Source: CAD feature listing. Evaluate the final solid. Frame: model axes, mm. Face numbers are marked on the shaded views. A direction names the side the tool comes from. Give positions to 0.01 mm unless a question says otherwise; leave off trailing zeros. Loops run counter-clockwise (first coordinate to the right, second up) from the corner with the lowest first, then second, coordinate; pieces in that order, holes last. Notation, with made-up numbers: (-27, 89.25) - (32, 89.25) arc R29 ccw to (32, 112.25) - close; hole circle Ø7 at (-25.5, 63). An arc over 180 degrees is marked (long way). Write each question's results on one line, items separated by ' | '. Start each with the question number.
(1) Cut plane D-D on z = 0.2. Return the cut outline in (x, y), then the cut area to 3 significant figures.
(2) Material intervals for line 1 along X through (y, z) = (23.25, -0.65); line 2 along Y through (x, z) = (-13, 0.3); line 3 along X through (y, z) = (21.25, 0.05), sorted ascending. Write a range as [from, to].
(3) Reachability of the marked faces 4, 5 and 6 from +Z, -Z, +X, -X, +Y, -Y: full face, straight path, thin tool, end or side. Return the list, or none.
(4) Cut plane A-A on z = -0.75. Return the cut outline in (x, y), then the cut area to 3 significant figures.
(5) Cut plane B-B on y = 25. Return the cut outline in (x, z), then the cut area to 3 significant figures.
(6) Cut plane C-C on x = -11. Return the cut outline in (y, z), then the cut area to 3 significant figures.
(7) Contact query for flat-ended pins moving along their axis: pin 1 (0.6 mm diameter, centred on x = -6.5, z = 0.5, fed in from -Y); pin 2 (4 mm diameter, centred on x = -8, y = 17, fed in from -Z); pin 3 (0.6 mm diameter, centred on y = 25, z = -1, fed in from -X). Output: stop coordinate, or through.
(8) Pull-direction query (X, two-part tool) for the marked faces 1, 2 and 3; classes: pulls with the +X half, pulls with the -X half, needs draft (parallel to the pull), parting line crosses it, or undercut.
Autodesk Fusion 360 part; units mm, degrees
sketch "Sketch1" plane through (0, 22, 0) normal (0, 1, 0) x (-1, 0, 0)
  line L0 (11.5698, 0.25) -> (15.3, 0.25)
  line L1 (15.3, 0.25) -> (15.3, -0.5)
  line L2 (15.3, -0.5) -> (15.6004, -0.5)
  line L3 (15.6004, -0.5) -> (15.6004, -1.2)
  line L4 (15.6004, -1.2) -> (16.0004, -1.2)
  line L5 (16.0004, -1.2) -> (16.0004, -0.5)
  line L6 (16.0004, -0.5) -> (16.3, -0.5)
  line L7 (16.3, -0.5) -> (16.3, 1.05)
  line L8 (16.3, 1.05) -> (5, 1.05)
  line L9 (11.5698, -1.2) -> (11.5698, 0.25)
  line L10 (11.5698, -0.6208) -> (11.2698, -0.6208) construction
  line L11 (11.2698, -0.5) -> (11.2698, -1.2)
  line L12 (11.2698, -0.5) -> (10.5698, -0.5)
  line L13 (10.5698, -0.5) -> (10.5698, -1.2)
  line L14 (10.5698, -0.678) -> (10.2698, -0.678) construction
  line L15 (10.2698, 1.05) -> (10.2698, -1.2)
  line L16 (10.2698, 1.05) -> (16.3, 1.05)
  line L17 (16.3, -0.5) -> (16.0004, -0.5)
  line L18 (16.0004, -1.2) -> (15.6004, -1.2)
  line L19 (15.6004, -0.5) -> (15.3, -0.5)
  line L20 (15.3, 0.25) -> (11.5698, 0.25)
  line L21 (11.5698, -1.2) -> (11.2698, -1.2)
  line L22 (11.5698, -1.2) -> (11.2698, -1.2)
  line L23 (11.2698, -0.5) -> (10.5698, -0.5)
  line L24 (10.5698, -1.2) -> (10.2698, -1.2)
  line L25 (10.2698, 1.05) -> (16.3, 1.05)
  line L26 (16.3, -0.5) -> (16.0004, -0.5)
  line L27 (16.0004, -1.2) -> (15.6004, -1.2)
  line L28 (15.6004, -0.5) -> (15.3, -0.5)
  line L29 (15.3, 0.25) -> (11.5698, 0.25)
  dimension "d14" = 0.3
  dimension "d15" = 0.7
  dimension "d16" = 0.3
extrude "Extrude1" add sketch "Sketch1" along normal blind 8.2 makes body 1
copy_body "Body->Comp1" bodies 1 removing the originals makes body 2 in component "Component"
move_face "OffsetFaces1" offset 0.3 1 faces at (-12.8132, 24.7333, 0.25) on bodies 2 in component "Component"
move_face "OffsetFaces2" offset -0.4 1 faces at (-12.2798, 27.4667, 1.05) on bodies 2 in component "Component"
move_face "OffsetFaces3" offset 3.3 1 faces at (-10.2698, 24.7333, 0.0333) on bodies 2 in component "Component"
move_face "OffsetFaces4" offset -3.3 1 faces at (-10.5698, 24.7333, -0.7333) on bodies 2 in component "Component"
move_face "OffsetFaces5" offset 3.3 1 faces at (-11.2698, 24.7333, -0.7333) on bodies 2 in component "Component"
move_face "OffsetFaces6" offset -3.3 1 faces at (-11.5698, 27.4667, -0.8167) on bodies 2 in component "Component"
move_face "OffsetFaces7" offset -4.2 1 faces at (-10.5132, 22, 0.4167) on bodies 2 in component "Component"
move_face "OffsetFaces8" offset -0.1 1 faces at (-8.2698, 28.8667, -0.4333) on bodies 2 in component "Component"
move_face "OffsetFaces9" offset 0.1 1 faces at (-7.9698, 27.5333, -0.7333) on bodies 2 in component "Component"
move_face "OffsetFaces10" offset 4.255 1 faces at (-10.4798, 26.2, 0.4167) on bodies 2 in component "Component"
move_face "OffsetFaces11" offset 0.3 1 faces at (-6.9698, 24.6967, 0.0333) on bodies 2 in component "Component"
move_face "OffsetFaces12" offset 0.3 1 faces at (-7.8698, 24.6967, -0.7333) on bodies 2 in component "Component"
move_face "OffsetFaces13" offset -0.3 1 faces at (-7.2698, 24.6967, -0.7333) on bodies 2 in component "Component"
move_face "OffsetFaces14" offset -0.3 1 faces at (-8.1698, 24.6967, -0.8167) on bodies 2 in component "Component"
move_face "OffsetFaces15" offset 2.77 1 faces at (-6.6698, 24.6967, 0.0333) on bodies 2 in component "Component"
move_face "OffsetFaces16" offset -2.77 1 faces at (-6.9698, 24.6967, -0.7333) on bodies 2 in component "Component"
move_face "OffsetFaces17" offset 2.77 1 faces at (-7.5698, 24.6967, -0.7333) on bodies 2 in component "Component"
move_face "OffsetFaces18" offset -2.77 1 faces at (-7.8698, 24.6967, -0.8167) on bodies 2 in component "Component"
move_face "OffsetFaces19" offset 6.445 1 faces at (-8.4332, 21.945, 0.4167) on bodies 2 in component "Component"
move_face "OffsetFaces20" offset 1.5 1 faces at (-12.1666, 20.4, 0.65) on bodies 2 in component "Component"
move_face "OffsetFaces21" offset -1.5 1 faces at (-8.4998, 20.4, -0.05) on bodies 2 in component "Component"
sketch "Sketch2" plane through (0, 0, 1.45) normal (0, 0, -1) x (1, 0, 0)
  line L0 (-5.0998, -15.5) -> (-15.3, -15.5)
  line L1 (-15.3, -15.5) -> (-15.3, -30.2)
  line L2 (-15.3, -30.2) -> (-5.0998, -30.2)
  line L3 (-5.0998, -30.2) -> (-5.0998, -15.5)
  line L4 (-5.0998, -15.5) -> (-5.0998, -26.3) construction
  line L5 (-5.0998, -26.3) -> (-15.3, -26.3)
  line L6 (-15.3, -26.3) -> (-15.3, -25.3)
  line L7 (-15.3, -25.3) -> (-5.0998, -25.3)
  line L8 (-5.0998, -25.3) -> (-5.0998, -26.3)
  dimension "d40" = 10.8
  dimension "d41" = 1
extrude "Extrude1'" add sketch "Sketch2" along normal blind 1.5 contours L1 L3 L5 L6 L7 L8 bodies 2 in component "Component"
move_face "OffsetFaces22" offset 6 1 faces at (-11.8999, 25.3, 0.95) on bodies 2 in component "Component"
move_face "OffsetFaces23" offset -6 1 faces at (-8.4998, 26.3, 0.45) on bodies 2 in component "Component"
move_face "OffsetFaces24" offset 0.3 1 faces at (-8.4998, 20.3, 0.45) on bodies 2 in component "Component"
move_face "OffsetFaces25" offset -0.3 1 faces at (-8.4998, 19.3, 0.45) on bodies 2 in component "Component"
move_face "OffsetFaces26" offset -0.6 1 faces at (-8.4998, 19.6, 0.45) on bodies 2 in component "Component"
sketch "Sketch3" plane through (0, 0, 1.45) normal (0, 0, -1) x (1, 0, 0)
  line L0 (-5.0998, -20.6) -> (-15.3, -20.6)
  line L1 (-15.3, -20.6) -> (-15.3, -30.2)
  line L2 (-15.3, -30.2) -> (-5.0998, -30.2)
  line L3 (-5.0998, -30.2) -> (-5.0998, -20.6)
  line L4 (-5.0998, -30.2) -> (-8.3998, -30.2)
  line L5 (-8.3998, -30.2) -> (-8.3998, -29.8)
  line L6 (-8.3998, -29.8) -> (-5.0998, -29.8)
  line L7 (-5.0998, -29.8) -> (-5.0998, -30.2)
  line L8 (-15.3, -30.2) -> (-10.9, -30.2)
  line L9 (-10.9, -30.2) -> (-10.9, -29.8)
  line L10 (-10.9, -29.8) -> (-15.3, -29.8)
  line L11 (-15.3, -29.8) -> (-15.3, -30.2)
  dimension "d49" = 3.3
  dimension "d50" = 0.4
  dimension "d51" = 4.4
  dimension "d52" = 0.4
extrude "Extrude2" add sketch "Sketch3" along normal blind 1.95 contours L2 L3 L4 L5 L6 L7 | L1 L2 L8 L9 L10 L11 bodies 2 in component "Component"
move_face "OffsetFaces27" offset 0.45 1 faces at (-11.8999, 20.3333, -0.05) on bodies 2 in component "Component"
move_face "OffsetFaces28" offset -1.4 1 faces at (-10.9, 30.0667, 0.8) on bodies 2 in component "Component"
move_face "OffsetFaces29" offset 1.4 1 faces at (-8.3998, 30.0667, 0.8) on bodies 2 in component "Component"
component "Component" placed x (1, 0, 0) y (0, 1, 0) z (0, 0, 1) at (0, 0, 0)
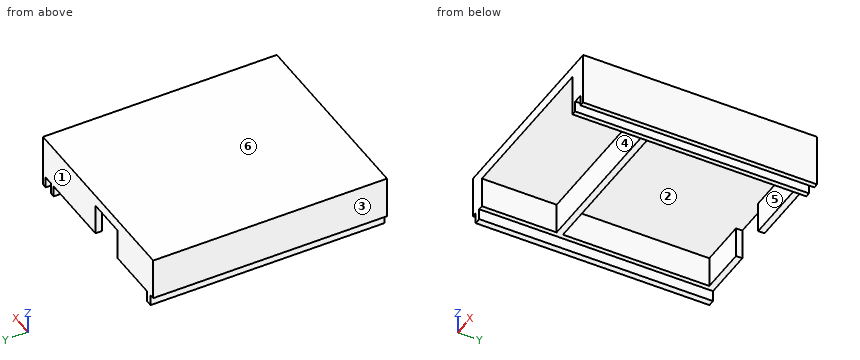
Ans:
1) outline: (-16.3, 15.5) - (-15.3, 15.5) - (-15.3, 20.2) - (-5.1, 20.2) - (-5.1, 15.5) - (-3.9, 15.5) - (-3.9, 30.2) - (-9.8, 30.2) - (-9.8, 29.8) - (-5.1, 29.8) - (-5.1, 20.6) - (-15.3, 20.6) - (-15.3, 29.8) - (-12.3, 29.8) - (-12.3, 30.2) - (-16.3, 30.2) - close | area: 39.5 mm^2
2) line 1: [-16, -15.6], [-5.1, -4.8], [-4.2, -3.9] | line 2: [20.2, 20.6], [29.8, 30.2] | line 3: [-16.3, -15.3], [-5.1, -3.9]
3) face 4: -Z, -Y | face 5: -Z | face 6: +Z, +X, -X, +Y, -Y
4) outline: (-16, 15.5) - (-15.6, 15.5) - (-15.6, 30.2) - (-16, 30.2) - close; (-5.1, 15.5) - (-4.8, 15.5) - (-4.8, 30.2) - (-5.1, 30.2) - close; (-4.2, 15.5) - (-3.9, 15.5) - (-3.9, 30.2) - (-4.2, 30.2) - close | area: 14.7 mm^2
5) outline: (-16.3, -0.5) - (-16, -0.5) - (-16, -1.2) - (-15.6, -1.2) - (-15.6, -0.5) - (-15.3, -0.5) - (-15.3, 1.45) - (-5.1, 1.45) - (-5.1, -1.2) - (-4.8, -1.2) - (-4.8, -0.5) - (-4.2, -0.5) - (-4.2, -1.2) - (-3.9, -1.2) - (-3.9, 2.15) - (-16.3, 2.15) - close | area: 13.7 mm^2
6) outline: (15.5, 1.45) - (20.2, 1.45) - (20.2, -0.5) - (20.6, -0.5) - (20.6, 1.45) - (30.2, 1.45) - (30.2, 2.15) - (15.5, 2.15) - close | area: 11.1 mm^2
7) pin 1: y = 20.2 | pin 2: z = 1.45 | pin 3: x = -16
8) face 1: needs draft | face 2: undercut | face 3: pulls with the -X half
